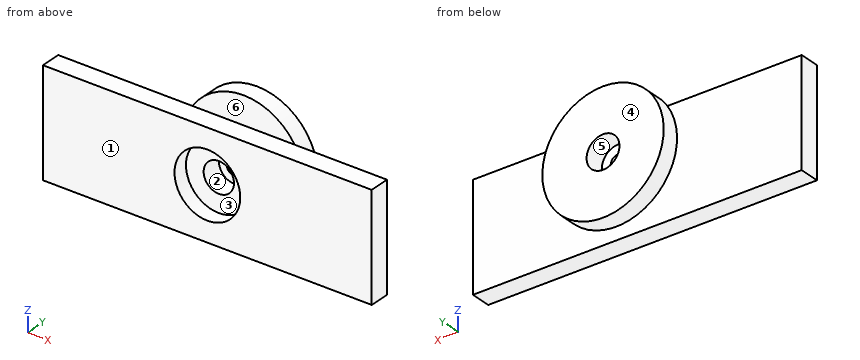
```python
from build123d import *

# Parameters (mm, degrees)
ESBO_O1_W                = 65
ESBO_O1_H                = 21
RESSALTO_EXTRUS_O3_DEPTH = 4
ESBO_O5_R                = 6.5
CORTE_EXTRUS_O2_DEPTH    = 3
ESBO_O6_R                = 3
CORTE_EXTRUS_O3_DEPTH    = 4
ESBO_O7_R                = 5
RESSALTO_EXTRUS_O4_DEPTH = 5.5
ESBO_O8_R                = 3.25
CORTE_EXTRUS_O4_DEPTH    = 0.5
ESBO_O10_R               = 3
CORTE_EXTRUS_O5_DEPTH    = 3
RESSALTO_EXTRUS_O5_START = 3.5
ESBO_O11_R               = 12
ESBO_O11_R_2             = 3.25
RESSALTO_EXTRUS_O5_DEPTH = 3.5
ESBO_O12_R               = 1.5
CORTE_EXTRUS_O6_DEPTH    = 5


with BuildPart() as part:
    # Esboço1 → Ressalto-extrusão3 (new body)
    with BuildSketch(Plane(origin=(0, 0, 0), x_dir=(1, 0, 0), z_dir=(0, 1, 0))):
        Rectangle(ESBO_O1_W, ESBO_O1_H)
    extrude(amount=RESSALTO_EXTRUS_O3_DEPTH)

    # Esboço5 → Corte-extrusão2 (cut)
    with BuildSketch(Plane.XZ):
        with Locations(Location((0, 0, 0), (0, 0, 270))):
            Circle(ESBO_O5_R)
    extrude(amount=-CORTE_EXTRUS_O2_DEPTH, mode=Mode.SUBTRACT)

    # Esboço6 → Corte-extrusão3 (cut)
    with BuildSketch(Plane.XZ.offset(-3)):
        with Locations(Location((0, 0, 0), (0, 0, 270))):
            Circle(ESBO_O6_R)
    extrude(amount=-CORTE_EXTRUS_O3_DEPTH, mode=Mode.SUBTRACT)

    # Esboço7 → Ressalto-extrusão4 (add)
    with BuildSketch(Plane(origin=(0, 4, 0), x_dir=(1, 0, 0), z_dir=(0, 1, 0))):
        with Locations(Location((0, 0, 0), (0, 0, 90))):
            Circle(ESBO_O7_R)
    extrude(amount=RESSALTO_EXTRUS_O4_DEPTH)

    # Esboço8 → Corte-extrusão4 (cut)
    with BuildSketch(Plane(origin=(0, 9.5, 0), x_dir=(1, 0, 0), z_dir=(0, 1, 0))):
        with Locations(Location((0, 0, 0), (0, 0, 270))):
            Circle(ESBO_O8_R)
    extrude(amount=-CORTE_EXTRUS_O4_DEPTH, mode=Mode.SUBTRACT)

    # Esboço10 → Corte-extrusão5 (cut)
    with BuildSketch(Plane.XZ.offset(-4)):
        with Locations(Location((0, 0, 0), (0, 0, 270))):
            Circle(ESBO_O10_R)
    extrude(amount=-CORTE_EXTRUS_O5_DEPTH, mode=Mode.SUBTRACT)

    # Esboço11 → Ressalto-extrusão5 (add)
    with BuildSketch(Plane(origin=(0, 9.5, 0), x_dir=(1, 0, 0), z_dir=(0, 1, 0)).offset(RESSALTO_EXTRUS_O5_START)):
        with Locations(Location((0, 0, 0), (0, 0, 270))):
            Circle(ESBO_O11_R)
        with Locations(Location((0, 0, 0), (0, 0, 270))):
            Circle(ESBO_O11_R_2, mode=Mode.SUBTRACT)
    extrude(amount=-RESSALTO_EXTRUS_O5_DEPTH)

    # Esboço12 → Corte-extrusão6 (cut)
    with BuildSketch(Plane(origin=(0, 9, 0), x_dir=(1, 0, 0), z_dir=(0, 1, 0))):
        with Locations(Location((0, 0, 0), (0, 0, 270))):
            Circle(ESBO_O12_R)
    extrude(amount=-CORTE_EXTRUS_O6_DEPTH, mode=Mode.SUBTRACT)


solid = part.part
```
Check sheet for the modelled part. Datum: model origin and axes. Units: mm. Face numbers are marked on the shaded views. A direction names the side the tool comes from. Coordinates: 2 decimals unless noted, no trailing zeros. Loops run counter-clockwise (first coordinate to the right, second up) from the corner with the lowest first, then second, coordinate; pieces in that order, holes last. Notation, with made-up numbers: M -15.75,12.5 L 38.25,12.5 A21 cw 38.25,39.5 Z; hole C -26.75,-14.5 d5. An arc over 180 degrees is marked long. Answer as a JSON object with one key per item and string values.
1. Sectioned sample at D-D on x = -22. Record the cut outline in (y, z), and give its area (3 significant figures).
Outcome:
{"outline": "M 0,-10.5 L 4,-10.5 L 4,10.5 L 0,10.5 Z", "area": "84.0 mm²"}
2. Sectioned sample at A-A on x = 0. Record the cut outline in (y, z).
Outcome:
{"outline": "M 0,-10.5 L 4,-10.5 L 4,-5 L 9.5,-5 L 9.5,-12 L 13,-12 L 13,-3.25 L 9,-3.25 L 9,-1.5 L 7,-1.5 L 7,-3 L 3,-3 L 3,-6.5 L 0,-6.5 Z; M 0,6.5 L 3,6.5 L 3,3 L 7,3 L 7,1.5 L 9,1.5 L 9,3.25 L 13,3.25 L 13,12 L 9.5,12 L 9.5,5 L 4,5 L 4,10.5 L 0,10.5 Z"}
3. Scan lines: L1, parallel to X at y = 4.05, z = 0; L2, parallel to X at y = 11.7, z = 0; L3, parallel to Y at x = 4, z = -9.75. Record each from-to range of solid material in increasing order. Write a range as from..to.
Outcome:
{"L1": "-5..-3, 3..5", "L2": "-12..-3.25, 3.25..12", "L3": "0..4, 9.5..13"}
4. Depth check by flat-ended pin: P1, Ø2, axis at y = 6, z = -9, coming from the -X side; P2, Ø6.5, axis at x = -1.5, z = -1.5, coming from the -Y side; P3, Ø1.2, axis at x = -11, y = 1.5, coming from the -Z side; P4, Ø2, axis at y = 7, z = 4, coming from the +X side. Enter the tip coordinate at first touch or a pass-through.
Outcome:
{"P1": "through", "P2": "y = 3", "P3": "z = -10.5", "P4": "x = 4"}
5. Sectioned sample at B-B on z = 0. Record the cut outline in (x, y).
Outcome:
{"outline": "M -32.5,0 L -6.5,0 L -6.5,3 L -3,3 L -3,7 L -1.5,7 L -1.5,9 L -3.25,9 L -3.25,13 L -12,13 L -12,9.5 L -5,9.5 L -5,4 L -32.5,4 Z; M 1.5,7 L 3,7 L 3,3 L 6.5,3 L 6.5,0 L 32.5,0 L 32.5,4 L 5,4 L 5,9.5 L 12,9.5 L 12,13 L 3.25,13 L 3.25,9 L 1.5,9 Z"}
6. Sectioned sample at C-C on y = 12.25. Record the cut outline in (x, z), and give its area (3 significant figures).
Outcome:
{"outline": "C 0,0 d24; hole C 0,0 d6.5", "area": "419 mm²"}
7. Access from +Z, -Z, +X, -X, +Y, -Y to the whole of each face (thin tool, end or side, straight path). Record for the marked faces 3, 4, 5 and 6.
Outcome:
{"face 3": "-Y", "face 4": "+Z, -Z, +X, -X, +Y", "face 5": "+Y", "face 6": "none"}
8. Release check for a two-part mould opening along Z. For the marked faces 1 and 2 record: pulls with the +Z half, pulls with the -Z half, needs draft (parallel to the pull), parting line crosses it, or undercut.
Outcome:
{"face 1": "needs draft", "face 2": "undercut"}
